Geometry: final body of the model. Coordinates: model frame, mm. A direction names the side the tool comes from. Round coordinates to 2 decimals unless told otherwise and drop trailing zeros. Loops run counter-clockwise (first coordinate to the right, second up) from the corner with the lowest first, then second, coordinate; pieces in that order, holes last. Notation, with made-up numbers: (-9.5, 89) - (12.5, 89) arc R26 cw to (12.5, 110) - close; hole circle Ø4 at (-29.75, 19). An arc over 180 degrees is marked (long way). Write item = value, one per line. Start each with the question number.
Item 1: Access query for faces 5 (the flat face through (-29, -6, -2)), 6 (the flat face through (-29, -1, -1)), 7 (the flat face through (0, 0, -3)). Directions: +Z, -Z, +X, -X, +Y, -Y. A direction counts if a zero-diameter tool reaches every point of the face in a straight line with its end or side. Return the directions, or none.
Item 2: First-contact query: pin 1 (1.5 mm diameter, centred on x = -19.5, z = -5, fed in from +Y); pin 2 (4.5 mm diameter, centred on y = -2.5, z = -6, fed in from +X); pin 3 (1.5 mm diameter, centred on x = -26, z = -1, fed in from -Y). Flat tips, straight axial feed; report the tip coordinate or a pass-through.
Item 3: Line query: line 1 (X direction, y = -3.25, z = -0.75); line 2 (Z direction, x = 36, y = -7.5); line 3 (Y direction, x = -34, z = -1.5). Output: solid intervals per line, ascending. Write a range as from..to.
Item 4: Draft query along X for faces 1 (the flat face through (19, 0.1, -3.3)), 2 (the flat face through (-39, 0, -1)), 3 (the flat face through (39, 0, -1)), 4 (the cylindrical face through (-19.52, 0.09, -6.31)). Return one class per face: pulls with the +X half, pulls with the -X half, needs draft (parallel to the pull), parting line crosses it, or undercut.
Item 5: Section A-A (x = 31.5). Return loops of the section in (y, z).
Item 6: Section D-D (y = 1.75). Return loops of the section in (x, z).
Item 7: Section B-B (y = -7.5). Return loops of the section in (x, z).
Item 8: Section C-C (z = -7.75). Return loops of the section in (x, y).
from build123d import *

# Parameters (mm, degrees)
SKETCH_W     = 78
SKETCH_H     = 20
PAD_DEPTH    = 2
SKETCH001_W  = 10
SKETCH001_H  = 5
PAD001_DEPTH = 5
SKETCH002_R  = 1.15
POCKET_DEPTH = 78.001
SKETCH003_W  = 3
SKETCH003_H  = 15
PAD002_DEPTH = 3.5
PAD003_DEPTH = 3
PAD004_DEPTH = 3
FILLET_R     = 1
SKETCH006_W  = 78
SKETCH006_H  = 2
PAD005_DEPTH = 3


with BuildPart() as part:
    # Sketch → Pad (new body)
    with BuildSketch(Plane.XY):
        Rectangle(SKETCH_W, SKETCH_H)
    extrude(amount=PAD_DEPTH)

    # Sketch001 (on Face5 of Pad) → Pad001 (join)
    with BuildSketch(Plane(origin=(0, 0, 0), x_dir=(1, 0, 0), z_dir=(0, 0, -1))):
        with Locations((34, 7.5)):
            Rectangle(SKETCH001_W, SKETCH001_H)
        with Locations((-34, 7.5)):
            Rectangle(SKETCH001_W, SKETCH001_H)
    extrude(amount=PAD001_DEPTH)

    # Sketch002 (on Face8 of Pad001) → Pocket (cut, through all)
    with BuildSketch(Plane.YZ.offset(39)):
        with Locations((-7.5, -2.5)):
            Circle(SKETCH002_R)
    extrude(amount=-POCKET_DEPTH, mode=Mode.SUBTRACT)

    # Sketch003 (on Face4 of Pocket) → Pad002 (join)
    with BuildSketch(Plane(origin=(0, 0, 0), x_dir=(1, 0, 0), z_dir=(0, 0, -1))):
        with Locations((37.5, -2.5)):
            Rectangle(SKETCH003_W, SKETCH003_H)
        with Locations((-37.5, -2.5)):
            Rectangle(SKETCH003_W, SKETCH003_H)
    extrude(amount=PAD002_DEPTH)

    # Sketch004 (on Face3 of Pad002) → Pad003 (join)
    with BuildSketch(Plane.YZ.offset(-21)):
        with BuildLine():
            Line((-6, 0), (6, 0))
            Line((6, 0), (6, -8.6))
            ThreePointArc((6, -8.6), (0, -6.308204), (-6, -8.6))
            Line((-6, 0), (-6, -8.6))
        make_face()
    extrude(amount=PAD003_DEPTH)

    # Sketch005 (on Face3 of Pad002) → Pad004 (join)
    with BuildSketch(Plane.YZ.offset(19)):
        with BuildLine():
            Line((-6, 0), (6, 0))
            Line((6, 0), (6, -8.6))
            ThreePointArc((6, -8.6), (0, -6.308204), (-6, -8.6))
            Line((-6, 0), (-6, -8.6))
        make_face()
    extrude(amount=PAD004_DEPTH)

    # Fillet
    fillet_edges = [part.edges().sort_by_distance(p)[0] for p in [
        (39, 10, 1),
        (39, 10, -1.75),
        (39, -10, -2.5),
        (39, -10, 1),
        (-39, -10, 1),
        (-39, -10, -2.5),
        (-39, 10, 1),
        (-39, 10, -1.75),
    ]]
    fillet(fillet_edges, radius=FILLET_R)

    # Sketch006 (on Face4 of Fillet) → Pad005 (join)
    with BuildSketch(Plane(origin=(0, 0, 0), x_dir=(1, 0, 0), z_dir=(0, 0, -1))):
        Rectangle(SKETCH006_W, SKETCH006_H)
        with Locations((0, -8)):
            Rectangle(SKETCH006_W, SKETCH006_H)
    extrude(amount=PAD005_DEPTH)


solid = part.part
Taken from the geometry:
q1.face_5 = -Z, -Y
q1.face_6 = -Z
q1.face_7 = -Z, +Y, -Y
q2.pin_1 = 6
q2.pin_2 = 22
q2.pin_3 = -1
q3.line_1 = -39..-36, -21..-18, 19..22, 36..39
q3.line_2 = -5..-3.65, -1.35..2
q3.line_3 = -10..-8.07, -6.93..-5, -1..1, 7..9
q4.face_1 = undercut
q4.face_2 = pulls with the -X half
q4.face_3 = pulls with the +X half
q4.face_4 = needs draft
q5.outline = (-10, -5) - (-5, -5) - (-5, 0) - (-1, 0) - (-1, -3) - (1, -3) - (1, 0) - (7, 0) - (7, -3) - (9, -3) - (9, 0) - (10, 0) - (10, 2) - (-10, 2) - close; hole circle Ø2.3 at (-7.5, -2.5)
q6.outline = (-39, -3.5) - (-36, -3.5) - (-36, 0) - (-21, 0) - (-21, -6.48) - (-18, -6.48) - (-18, 0) - (19, 0) - (19, -6.48) - (22, -6.48) - (22, 0) - (36, 0) - (36, -3.5) - (39, -3.5) - (39, 2) - (-39, 2) - close
q7.outline = (-39, -5) - (-29, -5) - (-29, -3.65) - (-39, -3.65) - close; (-39, -1.35) - (-29, -1.35) - (-29, 0) - (29, 0) - (29, -1.35) - (39, -1.35) - (39, 2) - (-39, 2) - close; (29, -5) - (39, -5) - (39, -3.65) - (29, -3.65) - close
q8.outline = (-21, -6) - (-18, -6) - (-18, -4.89) - (-21, -4.89) - close; (-21, 4.89) - (-18, 4.89) - (-18, 6) - (-21, 6) - close; (19, -6) - (22, -6) - (22, -4.89) - (19, -4.89) - close; (19, 4.89) - (22, 4.89) - (22, 6) - (19, 6) - close
